Geometry: see drawing. Coordinates: mm, zero at the bounding-box minimum. Round coordinates to 2 decimals unless told otherwise and drop trailing zeros. Order: outer loops, then holes, each group sorted by start corner. A loop starts at its lowest first (then second) coordinate and runs counter-clockwise, first axis right, second up. Notation, with made-up numbers: (42, -37) -> (54, -37) arc R20 cw to (54, -20) -> close; hole circle Ø4 at (31.25, -2). An arc over 180 degrees is marked (long way). Answer as CSV lines item,"result". Start each with the question number.
(1) Section query A-A (z = 4). Output: boundary loops of the cut face in (x, y) (1 decimal).
(2) Section query C-C (z = 19). Output: boundary loops of the cut face in (x, y) (1 decimal).
(3) Section query B-B (y = 1.25). Output: boundary loops of the cut face in (x, z) (1 decimal), plus the area to 3 significant figures.
(4) Contact query for a flat-ended pin moving along its axis: P1, Ø3, axis at x = 23.18, z = 3.49, coming from the -Y side. Output: stop coordinate, or through.
(5) Line query: line 1 along Z through (x, y) = (22, 0.95) (1 decimal); line 2 along X through (y, z) = (0.35, 17.75) (1 decimal); line 3 along X through (y, z) = (0.45, 3.75) (1 decimal). Output: solid intervals per line, ascending. Write a range as from..to.
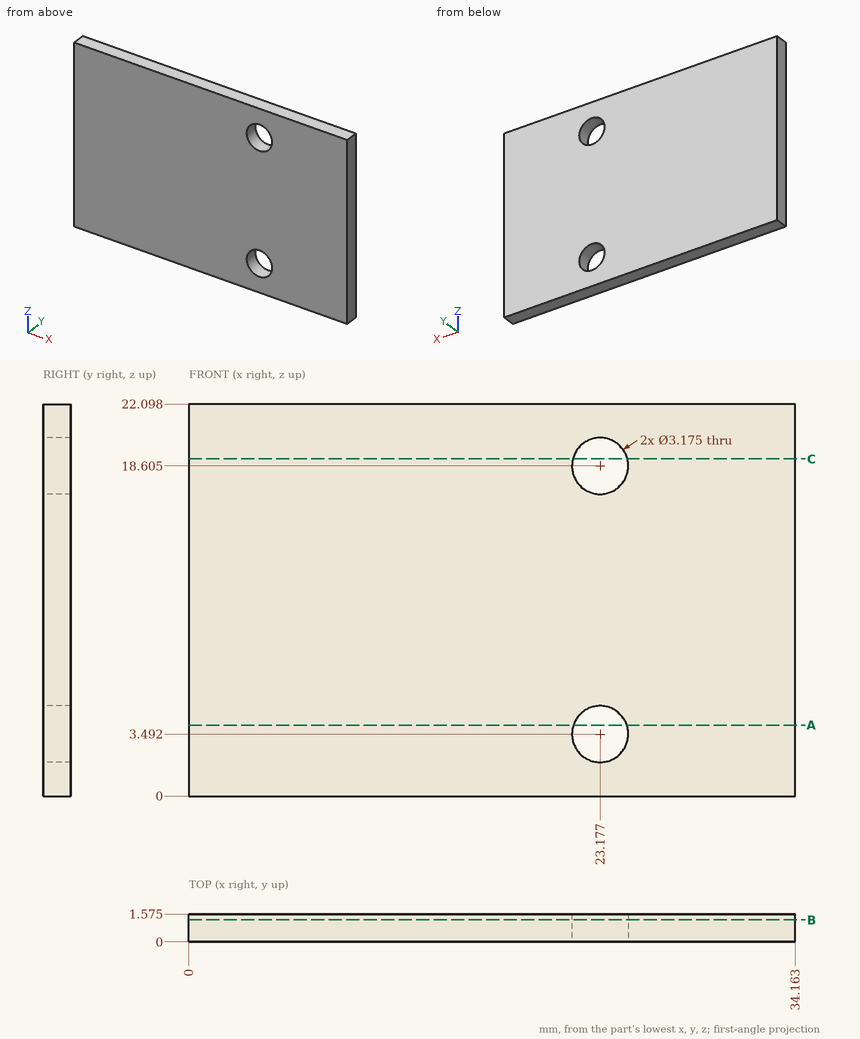
Answer block:
1,outline,"(0, 0) -> (21.7, 0) -> (21.7, 1.6) -> (0, 1.6) -> close; (24.7, 0) -> (34.2, 0) -> (34.2, 1.6) -> (24.7, 1.6) -> close"
2,outline,"(0, 0) -> (21.6, 0) -> (21.6, 1.6) -> (0, 1.6) -> close; (24.7, 0) -> (34.2, 0) -> (34.2, 1.6) -> (24.7, 1.6) -> close"
3,outline,"(0, 0) -> (34.2, 0) -> (34.2, 22.1) -> (0, 22.1) -> close; hole circle Ø3.2 at (23.2, 3.5); hole circle Ø3.2 at (23.2, 18.6)"
3,area,"739 mm2"
4,P1,"through"
5,line 1,"0..2.4, 4.6..17.5, 19.7..22.1"
5,line 2,"0..21.8, 24.5..34.2"
5,line 3,"0..21.6, 24.7..34.2"
